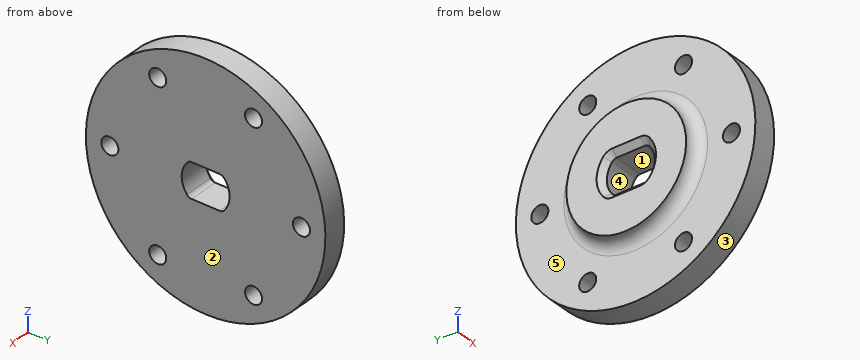
from build123d import *

# Parameters (mm, degrees)
SKETCH1_R           = 15.875
BOSS_EXTRUDE1_DEPTH = 3.175
SKETCH2_R           = 7.9375
BOSS_EXTRUDE2_DEPTH = 1.5875
CUT_EXTRUDE1_DEPTH  = 23.950221268
FILLET2_R           = 0.79375
CIRPATTERN1_COUNT   = 6
FILLET9_R           = 1.5875
CHAMFER1_SIZE       = 0.762


with BuildPart() as part:
    # Sketch1 → Boss-Extrude1 (new body)
    with BuildSketch(Plane(origin=(0, 0, 0), x_dir=(0, 0, -1), z_dir=(1, 0, 0))):
        Circle(SKETCH1_R)
    extrude(amount=BOSS_EXTRUDE1_DEPTH)

    # Sketch2 → Boss-Extrude2 (add)
    with BuildSketch(Plane.ZY):
        with Locations(Location((0, 0, 0), (0, 0, 180))):
            Circle(SKETCH2_R)
    extrude(amount=BOSS_EXTRUDE2_DEPTH)

    # Sketch3 → Cut-Extrude1 (cut, through all)
    with BuildSketch(Plane(origin=(3.175, 0, 0), x_dir=(0, 0, -1), z_dir=(1, 0, 0))):
        with BuildLine():
            Line((-2.286, 2.20336765), (-2.286, -2.20336765))
            ThreePointArc((-2.286, -2.20336765), (0, -3.175), (2.286, -2.20336765))
            Line((2.286, -2.20336765), (2.286, 2.20336765))
            ThreePointArc((2.286, 2.20336765), (0, 3.175), (-2.286, 2.20336765))
        make_face()
    extrude(amount=-CUT_EXTRUDE1_DEPTH, mode=Mode.SUBTRACT)

    # Fillet2
    fillet2_edges = [part.edges().sort_by_distance(p)[0] for p in [
        (0.79375, 2.20336765, 2.286),
        (0.79375, 2.20336765, -2.286),
        (0.79375, -2.20336765, -2.286),
        (0.79375, -2.20336765, 2.286),
    ]]
    fillet(fillet2_edges, radius=FILLET2_R)

    # Sketch5 → #4-40 Tapped Hole1 (revolve, cut)
    with BuildSketch(Plane(origin=(3.175, 12.7, 0), x_dir=(0, 0, -1), z_dir=(0, 1, 0))):
        Polygon((0, 0), (0, 8.299152758), (1.1303, 7.62), (1.1303, 0), align=None)
    f_4_40_tapped_hole1 = revolve(axis=Axis((9.525, 12.7, 0), (-1, 0, 0)), mode=Mode.SUBTRACT)

    # CirPattern1: #4-40 Tapped Hole1 ×6 about axis
    cirpattern1_axis = Axis((0, 0, 0), (1, 0, 0))
    for i in range(1, CIRPATTERN1_COUNT):
        add(f_4_40_tapped_hole1.rotate(cirpattern1_axis, i * 360 / CIRPATTERN1_COUNT), mode=Mode.SUBTRACT)

    # Fillet9
    fillet9_edges = [part.edges().sort_by_distance(p)[0] for p in [
        (0, 0, 7.9375),
    ]]
    fillet(fillet9_edges, radius=FILLET9_R - 0.0001)  # a hair under: the kernel refuses the full size

    # Chamfer1
    chamfer1_edges = [part.edges().sort_by_distance(p)[0] for p in [
        (-1.5875, 0, -2.286),
        (-1.5875, -3.175, 0),
        (-1.5875, 0, 2.286),
        (-1.5875, 3.175, 0),
        (-1.5875, -2.198617373, -2.208093398),
        (-1.5875, -2.198617373, 2.208093398),
        (-1.5875, 2.198617373, -2.208093398),
        (-1.5875, 2.198617373, 2.208093398),
    ]]
    chamfer(chamfer1_edges, length=CHAMFER1_SIZE)


solid = part.part
Design review of the part built by this model. Coordinates are the model's own, in mm. Face numbers are marked on the shaded views. A direction names the side the tool comes from. Give positions to 0.01 mm unless a question says otherwise; leave off trailing zeros. Write each loop counter-clockwise with the first axis right and the second up, starting at its lowest first coordinate (ties: lowest second). Pieces come first, ordered by that corner, then holes. Notation, with made-up numbers: M -18.5,79 L 17.5,79 A16 cw 17.5,103 Z; hole C 11.25,-2.5 d5. An arc over 180 degrees is marked long. Return JSON: item names as keys, results as strings. Group by question number.
Item 1: The part is to be moulded in two halves that separate along Y. For the marked faces 3, 4 and 5, say which applies: pulls with the +Y half, pulls with the -Y half, needs draft (parallel to the pull), parting line crosses it, or undercut.
Item 2: Take a section at D-D (y = -12). Give the boundary of the cut face in (x, z) (3 decimals), plus the area to 3 significant figures.
Item 3: Wall thickness on line 1 along Y through (x, z) = (0.75, 0) (3 decimals); line 2 along Z through (x, y) = (0.95, -12.7) (3 decimals); line 3 along Z through (x, y) = (2.25, -7): over which ranges is each line inside the solid? List them lowest first.
Item 4: Clearance check with flat-ended pins moving along their axes: pin 1 Ø1.8 at (y, z) = (-6.35, 11) entering from -X; pin 2 Ø2 at (x, z) = (1, 7) entering from +Y; pin 3 Ø2.5 at (y, z) = (-12.7, 0) entering from -X; pin 4 Ø2 at (x, z) = (0, 11.5) entering from -Y. State where each tip first meets the part, or that it passes through.
Item 5: Take a section at B-B (z = 0). Count the separate pieces of the cut face and the enclosed holes in it, plus the area to 3 significant figures.
Item 6: Tool access review of the marked faces 1 and 2: name each direction out of +Z, -Z, +X, -X, +Y, -Y from which nothing blocks a thin tool from reaching the whole face with its end or side.
Return value:
{
 "1": {"face 3": "parting line crosses it", "face 4": "undercut", "face 5": "needs draft"},
 "2": {"outline": "M 0,-10.393 L 3.175,-10.393 L 3.175,-0.887 L 0,-0.887 Z; M 0,0.887 L 3.175,0.887 L 3.175,10.393 L 0,10.393 Z", "area": "60.4 mm2"},
 "3": {"line 1": "y = -15.875 to -13.83, -11.57 to -3.175, 3.175 to 11.57, 13.83 to 15.875", "line 2": "z = -9.525 to -1.13, 1.13 to 9.525", "line 3": "z = -14.25 to -11.92, -10.07 to 10.07, 11.92 to 14.25"},
 "4": {"pin 1": "passes through", "pin 2": "stops at y = 14.7", "pin 3": "stops at x = 0", "pin 4": "stops at y = -11.91"},
 "5": {"separate pieces": "4", "enclosed holes": "0", "area": "81.9 mm2"},
 "6": {"face 1": "+X, -X", "face 2": "+Z, -Z, +X, +Y, -Y"}
}
